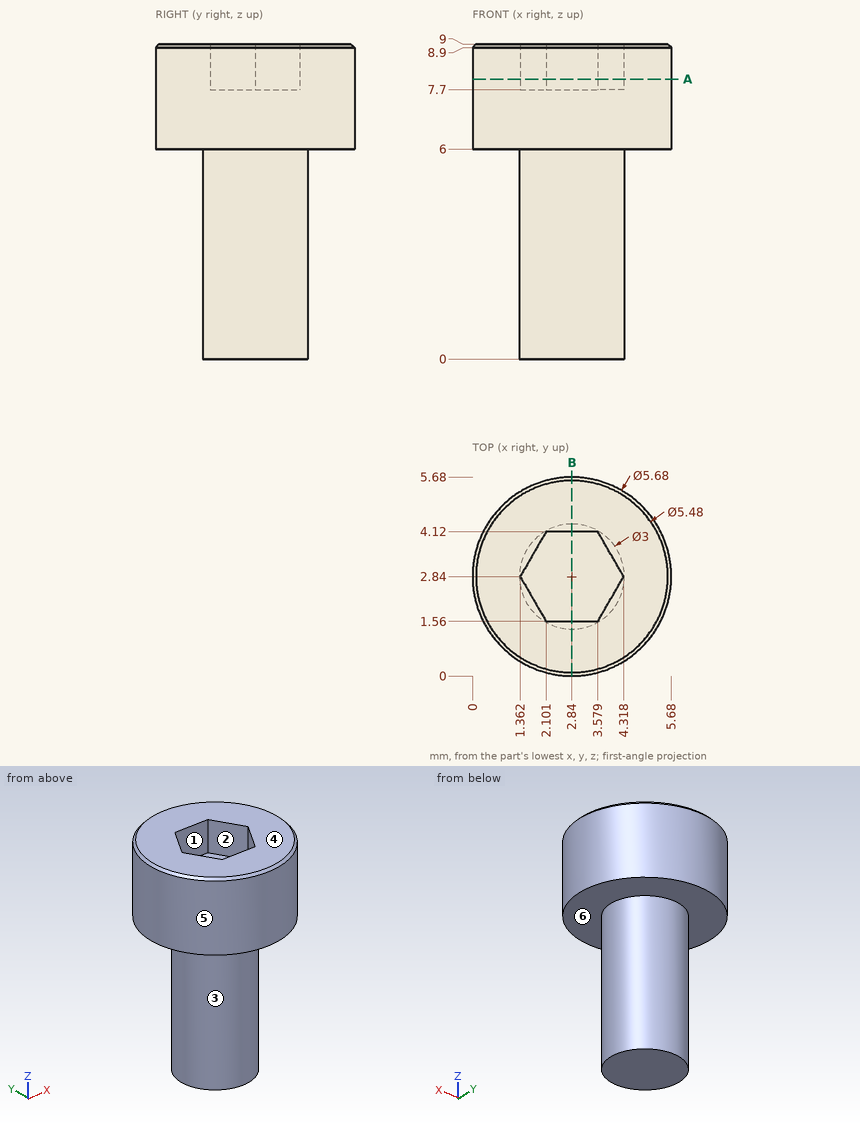
Part print with two shaded views. Sizes in mm from the minimum x, y, z corner. A direction names the side the tool comes from. Round coordinates to 2 decimals unless told otherwise and drop trailing zeros. Loops run counter-clockwise (first coordinate to the right, second up) from the corner with the lowest first, then second, coordinate; pieces in that order, holes last. Notation, with made-up numbers: M 12.5,57 L 20.5,57 A24 ccw 20.5,94 Z; hole C -12.5,3.25 d2. An arc over 180 degrees is marked long. Put each result on its own line as item: value. Start each with the question number.
Item 1: Cut at B-B (x = 2.84). List the corners of the cut face in (y, z).
Item 2: Mould opens along Y. For the marked faces 1, 2, 3 and 4 say: released by +Y, released by -Y, zero draft, split by the parting line, or undercut.
Item 3: 3-axis set-ups, long thin cutter, end or side, ignore diameter. For the marked faces 5 and 6: which of +Z, -Z, +X, -X, +Y, -Y reach the whole face in a straight line?
Item 4: Drop flat-ended pins along their axis: P1, Ø1, axis at x = 3.5, z = 6, coming from the -Y side; P2, Ø1.5, axis at y = 1.5, z = 3.5, coming from the -X side. Give the stop position or say it passes through.
Item 5: Cut at A-A (z = 8). List the corners of the cut face in (x, y).
Item 6: Drill centre lines: line 1 along Y through (x, z) = (2.95, 8.75); line 2 along Z through (x, y) = (1.85, 0.4); line 3 along Y through (x, z) = (3, 1.5). Where is each one in solid material? Low to high.
Answer block:
1. outline: M 0,6 L 1.34,6 L 1.34,0 L 4.34,0 L 4.34,6 L 5.68,6 L 5.68,8.9 L 5.58,9 L 4.12,9 L 4.12,7.7 L 1.56,7.7 L 1.56,9 L 0.1,9 L 0,8.9 Z
2. face 1: undercut
2. face 2: undercut
2. face 3: split by the parting line
2. face 4: zero draft
3. face 5: +Z, -Z
3. face 6: -Z
4. P1: y = 0
4. P2: x = 1.46
5. outline: C 2.84,2.84 d5.68; hole M 1.36,2.84 L 2.1,1.56 L 3.58,1.56 L 4.32,2.84 L 3.58,4.12 L 2.1,4.12 Z
6. line 1: 0 to 1.56, 4.12 to 5.68
6. line 2: 6 to 9
6. line 3: 1.35 to 4.33
